```python
from build123d import *

# Parameters (mm, degrees)
BOSS_EXTRUDE1_DEPTH     = 50.8
BOSS_EXTRUDE2_DEPTH     = 16.51
SKETCH4_W               = 127
SKETCH4_H               = 1.27
CUT_EXTRUDE1_DEPTH      = 102.6
F_1_4_CLEARANCE_HOLE1_D = 7.14248
FILLET1_R               = 5.08


with BuildPart() as part:
    # Sketch1 → Boss-Extrude1 (new body, symmetric)
    with BuildSketch(Plane.XY):
        with BuildLine():
            Line((55.88, 0), (63.5, 0))
            ThreePointArc((63.5, 0), (0, 63.5), (-63.5, 0))
            Line((-63.5, 0), (-55.88, 0))
            ThreePointArc((-55.88, 0), (0, 55.88), (55.88, 0))
        make_face()
    extrude(amount=BOSS_EXTRUDE1_DEPTH, both=True)

    # Sketch2 → Boss-Extrude2 (add)
    with BuildSketch(Plane(origin=(0, 0, -50.8), x_dir=(-1, 0, 0), z_dir=(0, 0, -1))):
        with BuildLine():
            Line((-63.5, 38.1), (-63.5, 0))
            ThreePointArc((-63.5, 0), (-60.241389426, 20.080463142), (-50.8, 38.1))
            Line((-50.8, 38.1), (-63.5, 38.1))
        make_face()
        with BuildLine():
            Line((63.5, 38.1), (50.8, 38.1))
            ThreePointArc((50.8, 38.1), (60.241389426, 20.080463142), (63.5, 0))
            Line((63.5, 0), (63.5, 38.1))
        make_face()
    boss_extrude2 = extrude(amount=-BOSS_EXTRUDE2_DEPTH)

    # Mirror1: Boss-Extrude2 across plane
    add(boss_extrude2.mirror(Plane.XY))

    # Sketch4 → Cut-Extrude1 (cut, through all)
    with BuildSketch(Plane.XY.offset(50.8)):
        with Locations((0, 0.635)):
            Rectangle(SKETCH4_W, SKETCH4_H)
    extrude(amount=-CUT_EXTRUDE1_DEPTH, mode=Mode.SUBTRACT)

    # 1/4 Clearance Hole1 (through all)
    with Locations(Plane(origin=(-57.15, 38.1, -44.45), x_dir=(0, 0, 1), z_dir=(0, 1, 0))):
        with Locations((0, 0), (0, 114.3), (88.9, 0), (88.9, 114.3)):
            Hole(F_1_4_CLEARANCE_HOLE1_D / 2)

    # Fillet1
    fillet1_edges = [part.edges().sort_by_distance(p)[0] for p in [
        (60.037562307, 20.681903014, 34.29),
        (-60.037562307, 20.681903014, 34.29),
        (-60.037562307, 20.681903014, -34.29),
        (60.037562307, 20.681903014, -34.29),
    ]]
    fillet(fillet1_edges, radius=FILLET1_R)


solid = part.part
```
Part model, mm, in its own coordinate system. A direction names the side the tool comes from. Coordinates: 2 decimals unless noted, no trailing zeros. Order: outer loops, then holes, each group sorted by start corner. A loop starts at its lowest first (then second) coordinate and runs counter-clockwise, first axis right, second up. Notation, with made-up numbers: (69.5, -29) -> (115.5, -29) arc R27 cw to (115.5, 7) -> close; hole circle Ø2 at (35.5, 37.25). An arc over 180 degrees is marked (long way). Put each result on its own line as item: value. Start each with the question number.
(1) Which spindle directions (+Z, -Z, +X, -X, +Y, -Y) get a long thin tool onto all of the face, cutting with end or side? Do faces 4 (the face through (-57, 38.1, 40)), 5 (the face through (1.379, 63.485, 0.711)), 6 (the face through (57, 38.1, -40)), 7 (the face through (-62, 35, 34.29)), 8 (the face through (62, 35, 34.29)). Say none if no direction does.
(2) Band-saw the part on D-D (x = 0). Give the cut face in (y, z).
(3) Pin check, flat tips, straight feed: pin 1 Ø14 at (x, z) = (55.5, 35) entering from +Y; pin 2 Ø8 at (x, z) = (-57.15, -44.45) entering from +Y; pin 3 Ø8 at (x, z) = (-44.5, 4.5) entering from -Y. Stop position of each tip, or through.
(4) Band-saw the part on C-C (y = 21). Count the separate pieces of the cut face and the enclosed holes in it, then the cut area to 3 significant figures.
(5) Band-saw the part on A-A (z = 44.45). Give the cut face in (x, y).
(6) Probe line 1 along Z through (x, y) = (57.15, 16); line 2 along X through (y, z) = (28, -44.45); line 3 along Z through (x, y) = (57.15, 29). List the from-to ranges inside material, lowest first. Write a range as [from, to].
(7) Mould opens along X. For faces 1 (the face through (-63.5, 19, 43)), 2 (the face through (-60.636, 19.427, 45.224)), 3 (the face through (-62, 35, -34.29)) say: pulls with the +X half, pulls with the -X half, needs draft (parallel to the pull), parting line crosses it, or undercut.
Determined:
1. face 4: +Z, -Z, -X, +Y
1. face 5: +Y
1. face 6: +Z, -Z, +X, +Y
1. face 7: -X, +Y
1. face 8: +X, +Y
2. outline: (55.88, -50.8) -> (63.5, -50.8) -> (63.5, 50.8) -> (55.88, 50.8) -> close
3. pin 1: stops at y = 40.99
3. pin 2: stops at y = 38.1
3. pin 3: stops at y = 27.75
4. separate pieces: 2
4. enclosed holes: 4
4. area: 1,750 mm²
5. outline: (-63.5, 1.27) -> (-60.72, 1.27) -> (-60.72, 38.1) -> (-63.5, 38.1) -> close; (-53.58, 15.87) arc R55.88 cw to (53.58, 15.87) -> (53.58, 38.1) -> (50.8, 38.1) arc R63.5 ccw to (-50.8, 38.1) -> (-53.58, 38.1) -> close; (60.72, 1.27) -> (63.5, 1.27) -> (63.5, 38.1) -> (60.72, 38.1) -> close
6. line 1: z = [-50.8, -48.02], [-40.88, 40.88], [48.02, 50.8]
6. line 2: x = [-63.5, -60.72], [-53.58, -48.36], [48.36, 53.58], [60.72, 63.5]
6. line 3: z = [-50.8, -48.02], [-40.88, -31.58], [31.58, 40.88], [48.02, 50.8]
7. face 1: pulls with the -X half
7. face 2: undercut
7. face 3: needs draft
